Geometry check sheet. Reference: the model listing, model coordinates, mm. A direction names the side the tool comes from. Round coordinates to 2 decimals unless told otherwise and drop trailing zeros. Write each loop counter-clockwise with the first axis right and the second up, starting at its lowest first coordinate (ties: lowest second). Pieces come first, ordered by that corner, then holes. Notation, with made-up numbers: (65, 72.5) -> (92, 72.5) arc R24 ccw to (92, 104.5) -> close; hole circle Ø9 at (-38.5, 63.5). An arc over 180 degrees is marked (long way). One line per question, with ' | ' between items.
```python
from build123d import *

# Parameters (mm, degrees)
SKETCH1_W            = 698.5
SKETCH1_H            = 84.582
BOSS_EXTRUDE1_DEPTH  = 34.925
SKETCH2_W            = 81.407
SKETCH2_H            = 31.75
CUT_EXTRUDE1_DEPTH   = 699.5
SKETCH3_W            = 698.5
SKETCH3_H            = 3.175
BOSS_EXTRUDE2_DEPTH  = 50.8
M2_CLEARANCE_HOLE1_D = 2.54
M5_CLEARANCE_HOLE1_D = 5.334
CHAMFER1_SIZE        = 3.175
FILLET1_R            = 0.762
FILLET2_R            = 3.937
SKETCH8_W            = 725.924928317
SKETCH8_H            = 218.216354959
CUT_EXTRUDE2_DEPTH   = 85.582


with BuildPart() as part:
    # Sketch1 → Boss-Extrude1 (new body)
    with BuildSketch(Plane(origin=(0, 57.816398039, 0), x_dir=(1, 0, 0), z_dir=(0, 1, 0))):
        with Locations((253.148031467, -103.269491579)):
            Rectangle(SKETCH1_W, SKETCH1_H)
    extrude(amount=-BOSS_EXTRUDE1_DEPTH)

    # Sketch2 → Cut-Extrude1 (cut, through all)
    with BuildSketch(Plane(origin=(602.398031467, 0, 0), x_dir=(0, 0, -1), z_dir=(1, 0, 0))):
        with Locations((-101.681991579, 41.941398039)):
            Rectangle(SKETCH2_W, SKETCH2_H)
    extrude(amount=-CUT_EXTRUDE1_DEPTH, mode=Mode.SUBTRACT)

    # Sketch3 → Boss-Extrude2 (add)
    with BuildSketch(Plane(origin=(0, 26.066398039, 0), x_dir=(-1, 0, 0), z_dir=(0, 1, 0))):
        with Locations((-253.148031467, 62.565991579)):
            Rectangle(SKETCH3_W, SKETCH3_H)
    extrude(amount=BOSS_EXTRUDE2_DEPTH)

    # M2 Clearance Hole1 (through all)
    with Locations(Plane(origin=(0, 26.066398039, 0), x_dir=(1, 0, 0), z_dir=(0, 1, 0))):
        with Locations((-96.101968533, -136.543491579), (-96.101968533, -69.995491579)):
            Hole(M2_CLEARANCE_HOLE1_D / 2)

    # M5 Clearance Hole1 (through all)
    with Locations(Plane(origin=(0, 0, 60.978491579), x_dir=(-1, 0, 0), z_dir=(0, 0, -1))):
        with Locations((-469.048031467, 64.928398039), (-481.748031467, 64.928398039), (-469.048031467, 39.528398039), (-481.748031467, 39.528398039), (-456.348031467, 39.528398039), (-443.648031467, 39.528398039), (-430.948031467, 39.528398039), (-418.248031467, 39.528398039), (-405.548031467, 39.528398039), (-392.848031467, 39.528398039), (-380.148031467, 39.528398039), (-367.448031467, 39.528398039), (-354.748031467, 39.528398039), (-342.048031467, 39.528398039), (-329.348031467, 39.528398039), (-316.648031467, 39.528398039), (-303.948031467, 39.528398039), (-291.248031467, 39.528398039), (-278.548031467, 39.528398039), (-265.848031467, 39.528398039), (-253.148031467, 39.528398039), (-240.448031467, 39.528398039), (-227.748031467, 39.528398039), (-215.048031467, 39.528398039), (-202.348031467, 39.528398039), (-189.648031467, 39.528398039), (-176.948031467, 39.528398039), (-164.248031467, 39.528398039), (-151.548031467, 39.528398039), (-138.848031467, 39.528398039), (-126.148031467, 39.528398039), (-113.448031467, 39.528398039), (-100.748031467, 39.528398039), (-88.048031467, 39.528398039), (-75.348031467, 39.528398039), (-62.648031467, 39.528398039), (-49.948031467, 39.528398039), (-37.248031467, 39.528398039), (-24.548031467, 39.528398039), (-11.848031467, 39.528398039), (0.851968533, 39.528398039), (13.551968533, 39.528398039), (26.251968533, 39.528398039), (38.951968533, 39.528398039), (51.651968533, 39.528398039), (64.351968533, 39.528398039), (77.051968533, 39.528398039), (89.751968533, 39.528398039), (-456.348031467, 64.928398039), (-443.648031467, 64.928398039), (-430.948031467, 64.928398039), (-418.248031467, 64.928398039), (-405.548031467, 64.928398039), (-392.848031467, 64.928398039), (-380.148031467, 64.928398039), (-367.448031467, 64.928398039), (-354.748031467, 64.928398039), (-342.048031467, 64.928398039), (-329.348031467, 64.928398039), (-316.648031467, 64.928398039), (-303.948031467, 64.928398039), (-291.248031467, 64.928398039), (-278.548031467, 64.928398039), (-265.848031467, 64.928398039), (-253.148031467, 64.928398039), (-240.448031467, 64.928398039), (-227.748031467, 64.928398039), (-215.048031467, 64.928398039), (-202.348031467, 64.928398039), (-189.648031467, 64.928398039), (-176.948031467, 64.928398039), (-164.248031467, 64.928398039), (-151.548031467, 64.928398039), (-138.848031467, 64.928398039), (-126.148031467, 64.928398039), (-113.448031467, 64.928398039), (-100.748031467, 64.928398039), (-88.048031467, 64.928398039), (-75.348031467, 64.928398039), (-62.648031467, 64.928398039), (-49.948031467, 64.928398039), (-37.248031467, 64.928398039), (-24.548031467, 64.928398039), (-11.848031467, 64.928398039), (0.851968533, 64.928398039), (13.551968533, 64.928398039), (26.251968533, 64.928398039), (38.951968533, 64.928398039), (51.651968533, 64.928398039), (64.351968533, 64.928398039), (77.051968533, 64.928398039), (89.751968533, 64.928398039), (-494.448031467, 64.928398039), (-494.448031467, 39.528398039), (-507.148031467, 64.928398039), (-507.148031467, 39.528398039), (-519.848031467, 64.928398039), (-519.848031467, 39.528398039), (-532.548031467, 64.928398039), (-532.548031467, 39.528398039), (-545.248031467, 64.928398039), (-545.248031467, 39.528398039), (-557.948031467, 64.928398039), (-557.948031467, 39.528398039), (-570.648031467, 64.928398039), (-570.648031467, 39.528398039), (-583.348031467, 64.928398039), (-583.348031467, 39.528398039), (-596.048031467, 64.928398039), (-596.048031467, 39.528398039)):
            Hole(M5_CLEARANCE_HOLE1_D / 2)

    # Chamfer1
    chamfer1_edges = [part.edges().sort_by_distance(p)[0] for p in [
        (-96.101968533, 57.816398039, 143.972991579),
        (-96.101968533, 76.866398039, 62.565991579),
        (602.398031467, 76.866398039, 62.565991579),
        (602.398031467, 57.816398039, 143.972991579),
    ]]
    chamfer(chamfer1_edges, length=CHAMFER1_SIZE)

    # Fillet1
    fillet1_edges = [part.edges().sort_by_distance(p)[0] for p in [
        (253.148031467, 26.066398039, 142.385491579),
        (253.148031467, 26.066398039, 64.153491579),
    ]]
    fillet(fillet1_edges, radius=FILLET1_R)

    # Fillet2
    fillet2_edges = [part.edges().sort_by_distance(p)[0] for p in [
        (253.148031467, 22.891398039, 60.978491579),
        (253.148031467, 22.891398039, 145.560491579),
    ]]
    fillet(fillet2_edges, radius=FILLET2_R)

    # Sketch8 → Cut-Extrude2 (cut, through all)
    with BuildSketch(Plane(origin=(0, 0, 60.978491579), x_dir=(-1, 0, 0), z_dir=(0, 0, -1))):
        with Locations((-330.360495626, 61.250645378)):
            Rectangle(SKETCH8_W, SKETCH8_H)
    extrude(amount=-CUT_EXTRUDE2_DEPTH, mode=Mode.SUBTRACT)


solid = part.part
```
(1) Access from +Z, -Z, +X, -X, +Y, -Y to the whole of each face (thin tool, end or side, straight path). Record for faces 1 (the cylindrical face through (-74.5, 40.3, 62.6)), 2 (the flat face through (-64, 46, 142.385)), 3 (the flat face through (-94.537, 56.207, 143.995)).
Resolved:
face 1: +Z, -Z | face 2: +X, -X, +Y | face 3: +Z, -X, +Y
(2) Sectioned sample at B-B on x = -85.5. Record the cut outline in (y, z).
Resolved:
outline: (22.89, 64.92) arc R3.94 ccw to (26.83, 60.98) -> (76.87, 60.98) -> (76.87, 64.15) -> (26.83, 64.15) arc R0.76 cw to (26.07, 64.92) -> (26.07, 141.62) arc R0.76 cw to (26.83, 142.39) -> (57.82, 142.39) -> (57.82, 145.56) -> (26.83, 145.56) arc R3.94 ccw to (22.89, 141.62) -> close
(3) Sectioned sample at D-D on x = -77.5. Record the cut outline in (y, z), then the cut area to 3 significant figures.
Resolved:
outline: (22.89, 64.92) arc R3.94 ccw to (26.83, 60.98) -> (36.9, 60.98) -> (36.9, 64.15) -> (26.83, 64.15) arc R0.76 cw to (26.07, 64.92) -> (26.07, 141.62) arc R0.76 cw to (26.83, 142.39) -> (36.9, 142.39) -> (36.9, 145.56) -> (26.83, 145.56) arc R3.94 ccw to (22.89, 141.62) -> close; (42.16, 60.98) -> (62.3, 60.98) -> (62.3, 64.15) -> (42.16, 64.15) -> close; (42.16, 142.39) -> (57.82, 142.39) -> (57.82, 145.56) -> (42.16, 145.56) -> close; (67.56, 60.98) -> (76.87, 60.98) -> (76.87, 64.15) -> (67.56, 64.15) -> close | area: 474 mm2
(4) Sectioned sample at C-C on z = 89.5. Record the cut outline in (x, y).
Resolved:
outline: (-96.1, 22.89) -> (-32.6, 22.89) -> (-32.6, 26.07) -> (-96.1, 26.07) -> close
(5) Material ranges on line 1 (Z direction, x = -83, y = 30); line 2 (Z direction, x = -92, y = 58); line 3 (Y direction, x = -75, z = 128.5), recorded low to high.
Resolved:
line 1: z = 60.98 to 64.15, 142.39 to 145.56 | line 2: z = 60.98 to 64.15 | line 3: y = 22.89 to 26.07
(6) Go/stop test with flat-tipped pins: pin 1 (3 mm diameter, centred on x = -64.35, y = 39.53, fed in from -Z); pin 2 (6 mm diameter, centred on x = -51.65, y = 64.93, fed in from +Z); pin 3 (4 mm diameter, centred on x = -88.5, z = 72.5, fed in from +Y). Record where each tip stops, or that it passes through.
Resolved:
pin 1: passes through | pin 2: stops at z = 64.15 | pin 3: stops at y = 26.07
(7) Draft check along X on faces 4 (the cylindrical face through (-63.907, 24.075, 62.101)), 5 (the cylindrical face through (-61.8, 40.3, 62.6)), 6 (the flat face through (-96.102, 24, 103)). Enter one of: +X half, -X half, draft (parallel to the pull), parting line (faces both ways), or undercut.
Resolved:
face 4: draft | face 5: undercut | face 6: -X half
(8) Sectioned sample at A-A on y = 28.5. Record the cut outline in (x, z), then the cut area to 3 significant figures.
Resolved:
outline: (-96.1, 60.98) -> (-32.6, 60.98) -> (-32.6, 64.15) -> (-96.1, 64.15) -> close; (-96.1, 142.39) -> (-32.6, 142.39) -> (-32.6, 145.56) -> (-96.1, 145.56) -> close | area: 403 mm2
